from build123d import *

# Parameters (mm, degrees)
SKETCH2_R           = 19.05
BOSS_EXTRUDE2_DEPTH = 9.525
CUT_EXTRUDE1_START  = -10.525
CUT_EXTRUDE1_DEPTH  = 11.525
CIRPATTERN1_COUNT   = 6
CUT_EXTRUDE2_DEPTH  = 10.525


with BuildPart() as part:
    # Sketch2 → Boss-Extrude2 (new body)
    with BuildSketch(Plane(origin=(0, 0, 0), x_dir=(1, 0, 0), z_dir=(0, 1, 0))):
        Circle(SKETCH2_R)
    extrude(amount=BOSS_EXTRUDE2_DEPTH)

    # Sketch3 → Cut-Extrude1 (cut)
    with BuildSketch(Plane(origin=(0, 9.525, 0), x_dir=(1, 0, 0), z_dir=(0, 1, 0)).offset(CUT_EXTRUDE1_START)):
        Polygon((0, 120.586851799), (0, 19.05), (0, 15.875), (10.530283709, 15.875), (112.067135509, 15.875), (250.709992792, 164.25655956), (138.642857283, 268.96841136), align=None)
    cut_extrude1 = extrude(amount=CUT_EXTRUDE1_DEPTH, mode=Mode.SUBTRACT)

    # CirPattern1: Cut-Extrude1 ×6 about axis
    cirpattern1_axis = Axis((0, 9.525, 0), (0, -1, 0))
    for i in range(1, CIRPATTERN1_COUNT):
        add(cut_extrude1.rotate(cirpattern1_axis, i * 360 / CIRPATTERN1_COUNT), mode=Mode.SUBTRACT)

    # Sketch4 → Cut-Extrude2 (cut, through all)
    with BuildSketch(Plane(origin=(0, 9.525, 0), x_dir=(1, 0, 0), z_dir=(0, 1, 0))):
        Polygon((0, 7.332348419), (-6.35, 3.666174209), (-6.35, -3.666174209), (0, -7.332348419), (6.35, -3.666174209), (6.35, 3.666174209), align=None)
    extrude(amount=-CUT_EXTRUDE2_DEPTH, mode=Mode.SUBTRACT)


solid = part.part
Work out the finished part from the listing and answer in its coordinate system (mm). A direction names the side the tool comes from. Give positions to 0.01 mm unless a question says otherwise; leave off trailing zeros. Loops run counter-clockwise (first coordinate to the right, second up) from the corner with the lowest first, then second, coordinate; pieces in that order, holes last. Notation, with made-up numbers: (-22.75, 6.5) - (19.25, 6.5) arc R8 ccw to (19.25, 13.5) - close; hole circle Ø6 at (75.25, -22.5). An arc over 180 degrees is marked (long way). Answer in a Markdown table with one row per item.
(1) Section C-C (z = -3) is taken. Give the vertices of the cut face in (x, y) (3 decimals).
Results list:
| item | result |
|---|---|
| outline | (-18.812, 0) - (-6.35, 0) - (-6.35, 9.525) - (-18.812, 9.525) - close; (6.35, 0) - (16.599, 0) - (16.599, 9.525) - (6.35, 9.525) - close |
(2) Flat-ended cylindrical pins translate along their axes: pin 1 Ø4 at (y, z) = (7, 13) entering from +X; pin 2 Ø5 at (x, y) = (5, 5.5) entering from -Z (3 decimals); pin 3 Ø2.5 at (y, z) = (2.5, 18) entering from -X. Find the tip coordinate at first contact, or state that the pin passes through.
Results list:
| item | result |
|---|---|
| pin 1 | stops at x = 11.98 |
| pin 2 | stops at z = -15.875 |
| pin 3 | stops at x = 0 |
(3) Consider L1, parallel to X at y = 4.25, z = 1.5; L2, parallel to Z at x = -5, y = 1.25 (3 decimals); L3, parallel to X at y = 4.75, z = -3. Determine where each line is inside the solid, lowest interval first. Write a range as [from, to].
Results list:
| item | result |
|---|---|
| L1 | x = [-17.46, -6.35], [6.35, 18.99] |
| L2 | z = [-18.382, -4.446], [4.446, 15.875] |
| L3 | x = [-18.81, -6.35], [6.35, 16.6] |
(4) A tool of negligible diameter and unlimited length cuts with its end or side. For faces 4 (the face through (0, 5, 17)), 5 (the face through (-16.344, 4.696, 3.442)), 6 (the face through (-15.14, 4.7, -8.74)), from which of +Z, -Z, +X, -X, +Y, -Y can it reach the whole face along a straight path? Write none if from no direction.
Results list:
| item | result |
|---|---|
| face 4 | +Z, -X, +Y, -Y |
| face 5 | -X, +Y, -Y |
| face 6 | -Z, +Y, -Y |
(5) Section D-D (x = 11.5) is taken. Give the vertices of the cut face in (y, z) (3 decimals), and give its area (3 significant figures).
Results list:
| item | result |
|---|---|
| outline | (0, -15.187) - (9.525, -15.187) - (9.525, 11.831) - (0, 11.831) - close |
| area | 257 mm² |
(6) Section B-B (x = 5) is taken. Give the vertices of the cut face in (y, z) (3 decimals), and give its area (3 significant figures).
Results list:
| item | result |
|---|---|
| outline | (0, -15.875) - (9.525, -15.875) - (9.525, -4.446) - (0, -4.446) - close; (0, 4.446) - (9.525, 4.446) - (9.525, 18.382) - (0, 18.382) - close |
| area | 242 mm² |
(7) For a pull along Z with two mould halves and no side action, classify faces 1 (the face through (6.35, 5, 0)), 2 (the face through (-18.22, 4.7, -5.56)), 3 (the face through (-13.924, 4.696, 13.001)) as pulls with the +Z half, pulls with the -Z half, needs draft (parallel to the pull), parting line crosses it, or undercut.
Results list:
| item | result |
|---|---|
| face 1 | undercut |
| face 2 | pulls with the -Z half |
| face 3 | pulls with the +Z half |
